```python
from build123d import *

# Parameters (mm, degrees)
F2_R     = 0.4
F3_R     = 2.49
F4_DEPTH = 1.4
F5_R     = 0.175


with BuildPart() as f1:
    # F0 (on Front) → F1 (revolve)
    with BuildSketch(Plane.XZ):
        with BuildLine():
            Line((-7, 0), (0, 0))
            Line((0, 0), (0, 1.573037))
            ThreePointArc((0, 1.573037), (-3.097478, 1.770684), (-6.144713, 2.360421))
            Line((-6.144713, 2.360421), (-7, 2.360421))
            Line((-7, 2.360421), (-7, 0))
        make_face()
    revolve(axis=Axis((0, 0, 0.786518), (0, 0, 1)))

    # F2
    f2_edges = [f1.edges().sort_by_distance(p)[0] for p in [
        (7, 0, 2.360421),
    ]]
    fillet(f2_edges, radius=F2_R)

    # F3 (on face) → F4 (join)
    with BuildSketch(Plane(origin=(0, 0, 0), x_dir=(1, 0, 0), z_dir=(0, 0, -1))):
        Circle(F3_R)
    extrude(amount=F4_DEPTH)

    # F5
    f5_edges = [f1.edges().sort_by_distance(p)[0] for p in [
        (-2.49, 0, -1.4),
        (-2.49, 0, 0),
        (7, 0, 0),
    ]]
    fillet(f5_edges, radius=F5_R)


solid = f1.part
```
CAD build for the part. Positions are in the model's coordinates, mm. A direction names the side the tool comes from. Give positions to 0.01 mm unless a question says otherwise; leave off trailing zeros. Loops run counter-clockwise (first coordinate to the right, second up) from the corner with the lowest first, then second, coordinate; pieces in that order, holes last. Notation, with made-up numbers: (-4, 56) - (48, 56) arc R25 cw to (48, 95) - close; hole circle Ø11 at (55.5, -31.5). An arc over 180 degrees is marked (long way). Put each result on its own line as item: value.
Q1. Probe line 1 along X through (y, z) = (0, -0.6); line 2 along Z through (x, y) = (-4.25, -5); line 3 along Z through (x, y) = (1, 1.75). List the from-to ranges inside material, lowest first.
Filled in:
line 1: x = -2.49 to 2.49
line 2: z = 0 to 2.36
line 3: z = -1.4 to 1.66
Q2. Tool access for faces 1 (the face through (0, 0, -1.4)), 2 (the face through (0, 3, 0)): list every direction of +Z, -Z, +X, -X, +Y, -Y with a clear straight run to the whole face (end or side of a thin tool).
Filled in:
face 1: -Z, +X, -X, +Y, -Y
face 2: -Z
Q3. Flat gauge pins, fed straight in: pin 1 (1.5 mm diameter, centred on y = -2.5, z = 1, fed in from -X); pin 2 (1 mm diameter, centred on y = -3, z = 2, fed in from -X); pin 3 (1 mm diameter, centred on x = 3, y = 0, fed in from +Z). Where does each tip first touch, or does it go through?
Filled in:
pin 1: stops at x = -6.78
pin 2: stops at x = -6.54
pin 3: stops at z = 1.83
Q4. Slice it at A-A (z = -0.6). Give the cut face in (x, y), plus the area to 3 significant figures.
Filled in:
outline: circle Ø4.98 at (0, 0)
area: 19.5 mm²
